For this review, take the finished solid that the model builds, in its own axes (mm). A direction names the side the tool comes from. Give positions to 0.01 mm unless a question says otherwise; leave off trailing zeros. Write each loop counter-clockwise with the first axis right and the second up, starting at its lowest first coordinate (ties: lowest second). Pieces come first, ordered by that corner, then holes.
1) Wall thickness on line 1 along Y through (x, z) = (0, 2); line 2 along Y through (x, z) = (0, 11); line 3 along Y through (x, z) = (11, 27.5): over which ranges is each line inside the solid? List them lowest first.
2) We need section C-C on z = 30. Give the boundary of the cut face in (x, y), and give its area (3 significant figures).
3) We need section A-A on y = 0. Give the number of separate pieces and of enclosed holes in the cut face, and give its area (3 significant figures).
4) Machinability: for faces 4 (the face through (20.61, -4.58, 19.85)), 5 (the face through (1.03, -51.56, 8.11)), which of the approach directions +Z, -Z, +X, -X, +Y, -Y give a long, thin tool a straight path to every point of the face, cutting with its end or side? Answer none if there is none.
5) We need section D-D on z = 12. Give the boundary of the cut face in (x, y) (1 decimal).
6) For P1, Ø5, axis at y = 19, z = 30, coming from the -X side; P2, Ø6, axis at y = 20.5, z = 5, coming from the -X side; P3, Ø9.5, axis at x = 0, y = -43.688, coming from the -Z side (3 decimals); P4, Ø5, axis at y = 5.5, z = 17.5, coming from the +X side, all flat-tipped, find the tip position at first contact; note any pin that passes through.
7) Draft analysis for pull direction Y (two halves, no side actions). For faces 1 (the face through (-1.03, 51.56, 8.11)), 2 (the face through (-46.612, -35.741, 7.32)), 3 (the face through (12, -12, 0)), state which applies: pulls with the +Y half, pulls with the -Y half, needs draft (parallel to the pull), parting line crosses it, or undercut.
from build123d import *

# Parameters (mm, degrees)
SKETCH1_R         = 58.7375
EXTRUDE1_DEPTH    = 16.002
SKETCH2_R         = 26.162
EXTRUDE2_DEPTH    = 19.812
SKETCH3_R         = 7.9375
EXTRUDE3_DEPTH    = 86.39732523
CIRPATTERN1_COUNT = 4
FILLET1_R         = 1.154545455


with BuildPart() as part:
    # Sketch1 → Extrude1 (new body)
    with BuildSketch(Plane.XY):
        Circle(SKETCH1_R)
    extrude(amount=EXTRUDE1_DEPTH)

    # Sketch2 → Extrude2 (add)
    with BuildSketch(Plane.XY.offset(16.002)):
        Circle(SKETCH2_R)
    extrude(amount=EXTRUDE2_DEPTH)

    # Sketch3 → Extrude3 (cut, through all)
    with BuildSketch(Plane.XY.offset(16.002)):
        with Locations((0, 43.688)):
            Circle(SKETCH3_R)
    extrude3 = extrude(amount=-EXTRUDE3_DEPTH, mode=Mode.SUBTRACT)

    # CirPattern1: Extrude3 ×4 about axis
    cirpattern1_axis = Axis((0, 0, 0), (0, 0, 1))
    for i in range(1, CIRPATTERN1_COUNT):
        add(extrude3.rotate(cirpattern1_axis, i * 360 / CIRPATTERN1_COUNT), mode=Mode.SUBTRACT)

    # Fillet1
    fillet1_edges = [part.edges().sort_by_distance(p)[0] for p in [
        (-58.7375, 0, 16.002),
        (-26.162, 0, 16.002),
        (-26.162, 0, 35.814),
    ]]
    fillet(fillet1_edges, radius=FILLET1_R)

    # Sketch4 → Cut-Revolve1 (revolve, cut)
    with BuildSketch(Plane(origin=(0, 0, 63.5), x_dir=(0, 0, -1), z_dir=(1, 0, 0))):
        Polygon((27.686, 21.209), (59.182, 21.0185), (59.182, 16.2306), (63.5, 16.2306), (63.5, 0), (27.686, 0), align=None)
    revolve(axis=Axis((0, 0, 0), (0, 0, 1)), mode=Mode.SUBTRACT)


solid = part.part
Results list:
1. line 1: y = -58.74 to -51.63, -35.75 to -16.23, 16.23 to 35.75, 51.63 to 58.74
1. line 2: y = -58.74 to -51.63, -35.75 to -21.06, 21.06 to 35.75, 51.63 to 58.74
1. line 3: y = -23.74 to -18.07, 18.07 to 23.74
2. outline: circle Ø52.32 at (0, 0); hole circle Ø42.35 at (0, 0)
2. area: 742 mm2
3. separate pieces: 4
3. enclosed holes: 0
3. area: 938 mm2
4. face 4: +Z
4. face 5: +Z, -Z
5. outline: circle Ø117.5 at (0, 0); hole circle Ø15.9 at (-43.7, 0); hole circle Ø42.1 at (0, 0); hole circle Ø15.9 at (0, -43.7); hole circle Ø15.9 at (0, 43.7); hole circle Ø15.9 at (43.7, 0)
6. P1: stops at x = -20.3
6. P2: stops at x = -56.07
6. P3: passes through
6. P4: stops at x = 58.51
7. face 1: undercut
7. face 2: parting line crosses it
7. face 3: needs draft
